```python
from build123d import *

# Parameters (mm, degrees)
BOSS_EXTRUDE1_DEPTH = 50
BOSS_EXTRUDE1_DRAFT = -20
SHELL3_T            = -5
BOSS_EXTRUDE3_DEPTH = 10
FILLET2_R           = 5
SKETCH12_R          = 1
CUT_EXTRUDE1_DEPTH  = 98.648600839


with BuildPart() as part:
    # Sketch3 → Boss-Extrude1 (with draft: the straight prism first)
    with BuildSketch(Plane(origin=(0, 0, 0), x_dir=(1, 0, 0), z_dir=(0, 1, 0))):
        Polygon((43.013605704, 4.982943342), (17.191447333, 39.742346919), (-25.822158371, 34.759403577), (-43.013605704, -4.982943342), (-17.191447333, -39.742346919), (25.822158371, -34.759403577), align=None)
    extrude(amount=-BOSS_EXTRUDE1_DEPTH)
    # Boss-Extrude1: the draft: its side faces are tilted about the plane it starts from
    boss_extrude1_sides = [part.faces().sort_by_distance(p)[0] for p in [
        (30.102526518, -25, -22.36264513),
        (-4.315355519, -25, -37.250875248),
        (-34.417882038, -25, -14.888230118),
        (-30.102526518, -25, 22.36264513),
        (4.315355519, -25, 37.250875248),
        (34.417882038, -25, 14.888230118),
    ]]
    draft(boss_extrude1_sides, Plane(origin=(0, 0, 0), x_dir=(1, 0, 0), z_dir=(0, 1, 0)), BOSS_EXTRUDE1_DRAFT)

    # Shell3
    shell3_openings = [part.faces().sort_by_distance(p)[0] for p in [
        (0, 0, 0),
    ]]
    offset(amount=SHELL3_T, openings=shell3_openings, kind=Kind.INTERSECTION)

    # Sketch11 → Boss-Extrude3 (add)
    with BuildSketch(Plane.XZ.offset(50)):
        Polygon((13.290828996, 17.890885893), (-8.848547182, 20.455638494), (-22.139376178, 2.564752601), (-13.290828996, -17.890885893), (8.848547182, -20.455638494), (22.139376178, -2.564752601), align=None)
    extrude(amount=BOSS_EXTRUDE3_DEPTH)

    # Fillet2
    fillet2_edges = [part.edges().sort_by_distance(p)[0] for p in [
        (22.139376178, -55, -2.564752601),
        (13.290828996, -55, 17.890885893),
        (-8.848547182, -55, 20.455638494),
        (-22.139376178, -55, 2.564752601),
        (-13.290828996, -55, -17.890885893),
        (8.848547182, -55, -20.455638494),
        (17.715102587, -60, 7.663066646),
        (2.221140907, -60, 19.173262194),
        (-15.49396168, -60, 11.510195548),
        (-17.715102587, -60, -7.663066646),
        (-2.221140907, -60, -19.173262194),
        (15.49396168, -60, -11.510195548),
    ]]
    fillet(fillet2_edges, radius=FILLET2_R)

    # Sketch12 → Cut-Extrude1 (cut, through all)
    with BuildSketch(Plane(origin=(-17.715102587, 0, -7.663066646), x_dir=(-0.39701946980837655, 0, 0.9178101876712176), z_dir=(-0.9178101876712177, 0, -0.3970194698083766))):
        with Locations((0, -55)):
            Circle(SKETCH12_R)
    extrude(amount=-CUT_EXTRUDE1_DEPTH, mode=Mode.SUBTRACT)


solid = part.part
```
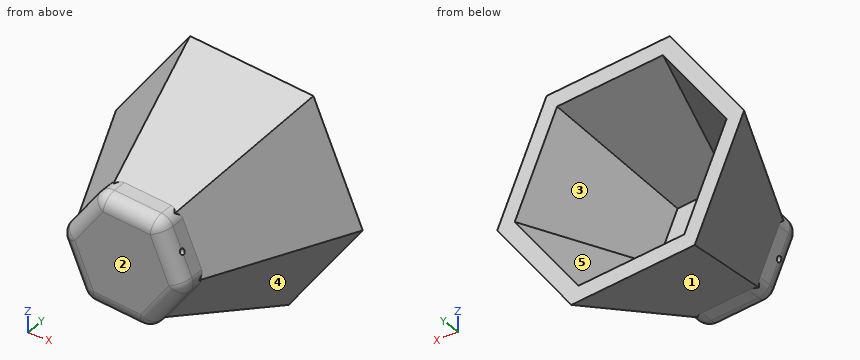
Here's how the part is built. I have some questions about the finished solid (model axes, mm). Face numbers are marked on the shaded views. A direction names the side the tool comes from. Coordinates: 2 decimals unless noted, no trailing zeros. Order: outer loops, then holes, each group sorted by start corner. A loop starts at its lowest first (then second) coordinate and runs counter-clockwise, first axis right, second up.
Item 1: If we section it at A-A, the plane y = -24: List the corners of the cut face in (x, z) for me.
Response values:
outline: (-32.99, 3.82) - (-19.81, -26.66) - (13.19, -30.48) - (32.99, -3.82) - (19.81, 26.66) - (-13.19, 30.48) - close; hole (-26.89, 3.12) - (-16.14, -21.73) - (10.75, -24.85) - (26.89, -3.12) - (16.14, 21.73) - (-10.75, 24.85) - close
Item 2: If we section it at D-D, the plane y = -39: List the corners of the cut face in (x, z) for me.
Response values:
outline: (-26.73, 3.1) - (-16.05, -21.6) - (10.68, -24.7) - (26.73, -3.1) - (16.05, 21.6) - (-10.68, 24.7) - close; hole (-20.63, 2.39) - (-12.38, -16.67) - (8.24, -19.06) - (20.63, -2.39) - (12.38, 16.67) - (-8.24, 19.06) - close
Item 3: Which directions (+Z, -Z, +X, -X, +Y, -Y) give clear straight access to the entire face, cutting with the end or side of a thin tool? Please do the marked faces 4 and 5.
Response values:
face 4: -Z, +X, -Y
face 5: +Y
Item 4: If we section it at C-C, the plane x = -27: List the corners of the cut face in (y, z) for me, then the cut area to 3 significant figures.
Response values:
outline: (-38.36, 3.13) - (0, -32.04) - (0, -18.63) - (-23.74, 3.13) - (0, 17.62) - (0, 26.54) - close
area: 693 mm2
Item 5: Thinking about a two-plate mould opening in Z: for the marked faces 1, 2 and 3, which applies, pulls with the +Z half, pulls with the -Z half, needs draft (parallel to the pull), parting line crosses it, or undercut?
Response values:
face 1: pulls with the -Z half
face 2: needs draft
face 3: undercut
Item 6: I'm going to push flat-ended pins straight in: pin 1 Ø5 at (y, z) = (-7.5, -24) entering from +X; pin 2 Ø3 at (x, y) = (-20, -36) entering from -Z; pin 3 Ø1.5 at (y, z) = (-10.5, 27.5) entering from +X. Where does each tip first touch, or does it pass through?
Response values:
pin 1: stops at x = 27.66
pin 2: stops at z = -18.95
pin 3: stops at x = 25.24
Item 7: If we section it at B-B, the plane z = 31.5: List the corners of the cut face in (x, y) for me, then the cut area to 3 significant figures.
Response values:
outline: (-23.31, 0) - (-13.63, -21.37) - (23.4, -9.66) - (27.23, 0) - (7.72, 0) - (-13.63, -6.75) - (-16.69, 0) - close
area: 614 mm2
Item 8: I need wall thicknesses on probe 1 along Y at (x, z) = (2, 1); probe 2 along X at (y, z) = (-18, 5); probe 3 along Z at (x, y) = (-22, -11). Which ranges of each line are inside material? Lowest first, please.
Response values:
probe 1: y = -60 to -55.99, -54.01 to -45
probe 2: x = -34.84 to -28.21, 25.76 to 31.56
probe 3: z = -31.17 to -20.11, 17.63 to 26.56
